Autodesk Inventor part; units mm, degrees
ref_plane "YZ Plane" through (0, 0, 0) normal (1, 0, 0) x (0, 1, 0)
ref_plane "XZ Plane" through (0, 0, 0) normal (0, 1, 0) x (-1, 0, 0)
ref_plane "XY Plane" through (0, 0, 0) normal (0, 0, 1) x (1, 0, 0)
sketch "Body Outline" plane through (0, 0, 0) normal (0, 1, 0) x (-1, 0, 0)
  line L0 (37.5, -6) -> (-37.5, -6)
  line L1 (-37.5, -6) -> (-37.5, 6)
  line L2 (-37.5, 6) -> (37.5, 6)
  line L3 (37.5, 6) -> (37.5, -6)
  point P0 (0, 0)
  dimension "d0" = 75
  dimension "d1" = 37.5
  dimension "d2" = 12
  dimension "d3" = 6
extrude "Body" add sketch "Body Outline" along normal blind 6
sketch "Clamp Cutout Outline" plane through (37.5, 0, 6) normal (1, 0, 0) x (0, 0, -1)
  line L0 (2, 7.3) -> (10, 7.3)
  line L1 (10, 7.3) -> (10, 5.3)
  line L2 (10, 5.3) -> (2, 5.3)
  line L3 (2, 5.3) -> (2, 7.3)
  line L4 (0, 6) -> (12, 6)
  line L5 (0, 0) -> (0, 6)
  line L6 (12, 0) -> (12, 6)
  point P0 (6, 0)
  dimension "d6" = 0.7
  dimension "d7" = 2
  dimension "d8" = 2
  dimension "d9" = 2
extrude "Clamp Cutout" cut sketch "Clamp Cutout Outline" along normal through all both and the other way through all
sketch "Fastening Hole Positions" plane through (0, 0, 0) normal (0, -1, 0) x (1, 0, 0)
  point P0 (0, 0)
  point P1 (20, 0)
  point P2 (0, 0)
  point P3 (-20, 0)
  dimension "d12" = 20
  dimension "d13" = 20
  dimension "d14" = 0
  dimension "d15" = 0
  dimension "d16" = 0
  dimension "d17" = 0
hole "Fastening Holes" at (20, 0, 0) at (0, 0, 0) at (-20, 0, 0) direction (0, 1, 0) diameter 5.2 end through all countersink diameter 11 countersink angle 90
equation "\"d8\" = d7"
properties part number "LR Small Clamp" material "Aluminum 6061"
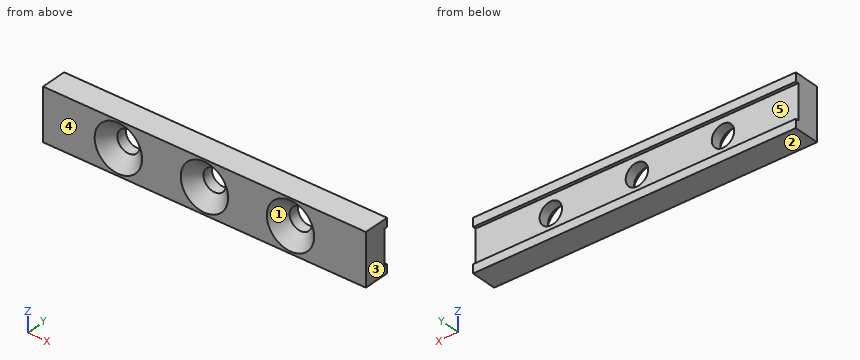
The listing builds one solid part. Answer for the finished solid, in the listing's coordinates (mm). Face numbers are marked on the shaded views. A direction names the side the tool comes from. Round coordinates to 2 decimals unless told otherwise and drop trailing zeros. Loops run counter-clockwise (first coordinate to the right, second up) from the corner with the lowest first, then second, coordinate; pieces in that order, holes last.
Q1. Section D-D, the plane x = -7.5 is taken. Determine the outline of the cut face in (y, z), then the cut area to 3 significant figures.
Q2. Given pin 1 Ø3 at (x, z) = (-20, 0) entering from +Y; pin 2 Ø6.5 at (x, z) = (-12, -0.5) entering from +Y, each flat-ended and moving along its own axis, determine where each tip first touches the part or whether it passes through.
Q3. Section C-C, the plane x = 0 is taken. Determine the outline of the cut face in (y, z), then the cut area to 3 significant figures.
Q4. Find the intervals of material crossed by line 1 (X direction, y = 4.55, z = 0); line 2 (Z direction, x = 20, y = 4.45); line 3 (X direction, y = 1.3, z = -1.5), in increasing order.
Q5. For a pull along Z with two mould halves and no side action, classify the marked faces 1, 2 and 3 as released by +Z, released by -Z, zero draft, split by the parting line, or undercut.
Q6. Section A-A, the plane y = 1.25 is taken. Determine the outline of the cut face in (x, z), then the cut area to 3 significant figures.
Q7. Which of the six approach directions +Z, -Z, +X, -X, +Y, -Y give full straight-line access (tool end or side, diameter ignored) to the marked faces 4 and 5?
Q8. Section B-B, the plane z = 0 is taken. Determine the outline of the cut face in (x, y), then the cut area to 3 significant figures.
Completed:
1. outline: (0, -6) - (6, -6) - (6, -4) - (5.3, -4) - (5.3, 4) - (6, 4) - (6, 6) - (0, 6) - close
1. area: 66.4 mm2
2. pin 1: passes through
2. pin 2: stops at y = 5.3
3. outline: (0, -6) - (6, -6) - (6, -4) - (5.3, -4) - (5.3, -2.6) - (2.9, -2.6) - (0, -5.5) - close; (0, 5.5) - (2.9, 2.6) - (5.3, 2.6) - (5.3, 4) - (6, 4) - (6, 6) - (0, 6) - close
3. area: 30.4 mm2
4. line 1: x = -37.5 to -22.6, -17.4 to -2.6, 2.6 to 17.4, 22.6 to 37.5
4. line 2: z = -6 to -2.6, 2.6 to 6
4. line 3: x = -37.5 to -23.92, -16.08 to -3.92, 3.92 to 16.08, 23.92 to 37.5
5. face 1: undercut
5. face 2: released by -Z
5. face 3: zero draft
6. outline: (-37.5, -6) - (37.5, -6) - (37.5, 6) - (-37.5, 6) - close; hole circle Ø8.5 at (-20, 0); hole circle Ø8.5 at (0, 0); hole circle Ø8.5 at (20, 0)
6. area: 730 mm2
7. face 4: +Z, -Z, +X, -X, -Y
7. face 5: +X, -X, +Y
8. outline: (-37.5, 0) - (-25.5, 0) - (-22.6, 2.9) - (-22.6, 5.3) - (-37.5, 5.3) - close; (-17.4, 2.9) - (-14.5, 0) - (-5.5, 0) - (-2.6, 2.9) - (-2.6, 5.3) - (-17.4, 5.3) - close; (2.6, 2.9) - (5.5, 0) - (14.5, 0) - (17.4, 2.9) - (17.4, 5.3) - (2.6, 5.3) - close; (22.6, 2.9) - (25.5, 0) - (37.5, 0) - (37.5, 5.3) - (22.6, 5.3) - close
8. area: 290 mm2
